Check sheet for the modelled part. Datum: model origin and axes. Units: mm. Face numbers are marked on the shaded views. Give positions to 0.01 mm unless a question says otherwise; leave off trailing zeros. Write each loop counter-clockwise with the first axis right and the second up, starting at its lowest first coordinate (ties: lowest second). Pieces come first, ordered by that corner, then holes. Notation, with made-up numbers: (18.5, 40) -> (60.5, 40) arc R21 cw to (60.5, 63) -> close; hole circle Ø1 at (-2, 72). An arc over 180 degrees is marked (long way). Return JSON: item names as keys, results as strings.
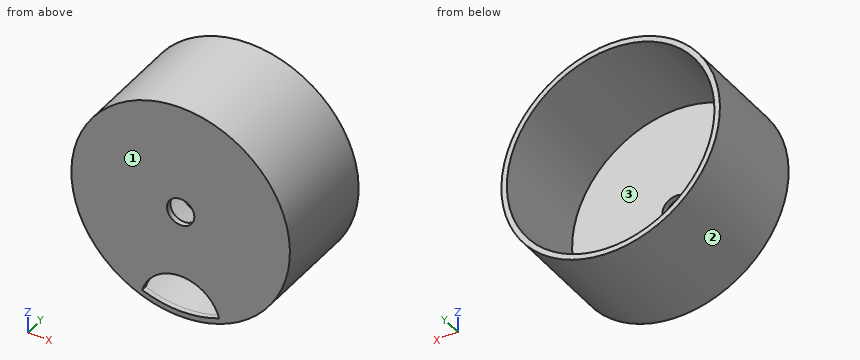
from build123d import *

# Parameters (mm, degrees)
SKETCH1_R           = 40
BOSS_EXTRUDE1_DEPTH = 40
SKETCH2_R           = 38
CUT_EXTRUDE1_DEPTH  = 38
CUT_EXTRUDE2_DEPTH  = 38
SKETCH4_R           = 5
CUT_EXTRUDE3_DEPTH  = 38


with BuildPart() as part:
    # Sketch1 → Boss-Extrude1 (new body)
    with BuildSketch(Plane(origin=(0, 0, 0), x_dir=(1, 0, 0), z_dir=(0, 1, 0))):
        with Locations(Location((0, 0, 0), (0, 0, 270))):
            Circle(SKETCH1_R)
    extrude(amount=BOSS_EXTRUDE1_DEPTH)

    # Sketch2 → Cut-Extrude1 (cut)
    with BuildSketch(Plane(origin=(0, 40, 0), x_dir=(1, 0, 0), z_dir=(0, 1, 0))):
        with Locations(Location((0, 0, 0), (0, 0, 270))):
            Circle(SKETCH2_R)
    extrude(amount=-CUT_EXTRUDE1_DEPTH, mode=Mode.SUBTRACT)

    # Sketch3 → Cut-Extrude2 (cut)
    with BuildSketch(Plane(origin=(0, 2, 0), x_dir=(1, 0, 0), z_dir=(0, 1, 0))):
        with BuildLine():
            ThreePointArc((-14.076066703, 35.296803626), (0, 24.534862453), (14.076066703, 35.296803626))
            ThreePointArc((14.076066703, 35.296803626), (0, 38), (-14.076066703, 35.296803626))
        make_face()
    extrude(amount=-CUT_EXTRUDE2_DEPTH, mode=Mode.SUBTRACT)

    # Sketch4 → Cut-Extrude3 (cut)
    with BuildSketch(Plane(origin=(0, 2, 0), x_dir=(1, 0, 0), z_dir=(0, 1, 0))):
        with Locations(Location((0, 0, 0), (0, 0, 270))):
            Circle(SKETCH4_R)
    extrude(amount=-CUT_EXTRUDE3_DEPTH, mode=Mode.SUBTRACT)


solid = part.part
(1) Depth check by flat-ended pin: pin 1 Ø12 at (x, y) = (-0.5, 9.5) entering from -Z; pin 2 Ø6 at (x, y) = (27, 29) entering from +Z; pin 3 Ø4 at (x, y) = (-10.5, 19) entering from -Z; pin 4 Ø2 at (y, z) = (7.5, 26.5) entering from +X. Enter the tip coordinate at first touch or a pass-through.
Reply:
{"pin 1": "z = -40", "pin 2": "z = 32", "pin 3": "z = -39.09", "pin 4": "x = 30.82"}
(2) Cross-section at D-D on z = -12.5. Enter the section's corners in (x, y), then the cut area to 3 significant figures.
Reply:
{"outline": "(-38, 0) -> (38, 0) -> (38, 40) -> (35.89, 40) -> (35.89, 2) -> (-35.89, 2) -> (-35.89, 40) -> (-38, 40) -> close", "area": "312 mm^2"}
(3) Cross-section at A-A on z = 0. Enter the section's corners in (x, y).
Reply:
{"outline": "(-40, 0) -> (-5, 0) -> (-5, 2) -> (-38, 2) -> (-38, 40) -> (-40, 40) -> close; (5, 0) -> (40, 0) -> (40, 40) -> (38, 40) -> (38, 2) -> (5, 2) -> close"}
(4) Thickness scan on L1, parallel to X at y = 29.5, z = 0; L2, parallel to Y at x = 6, z = -5; L3, parallel to X at y = 37.5, z = 33.5. Record the ranges inside material, lowest first.
Reply:
{"L1": "-40 to -38, 38 to 40", "L2": "0 to 2", "L3": "-21.86 to -17.94, 17.94 to 21.86"}
(5) Cross-section at B-B on x = 0. Enter the section's corners in (y, z), then the cut area to 3 significant figures.
Reply:
{"outline": "(0, -40) -> (40, -40) -> (40, -38) -> (0, -38) -> close; (0, -24.53) -> (2, -24.53) -> (2, -5) -> (0, -5) -> close; (0, 5) -> (2, 5) -> (2, 38) -> (40, 38) -> (40, 40) -> (0, 40) -> close", "area": "265 mm^2"}
(6) Cross-section at C-C on y = 30.5. Enter the section's corners in (x, z), then the cut area to 3 significant figures.
Reply:
{"outline": "circle Ø80 at (0, 0); hole circle Ø76 at (0, 0)", "area": "490 mm^2"}
(7) Release check for a two-part mould opening along X. For the marked faces 1, 2 and 3 record: pulls with the +X half, pulls with the -X half, needs draft (parallel to the pull), parting line crosses it, or undercut.
Reply:
{"face 1": "needs draft", "face 2": "parting line crosses it", "face 3": "undercut"}
